Check sheet for the drawn part. Datum: minimum x, y, z corner. Units: mm. A direction names the side the tool comes from. Give positions to 0.01 mm unless a question says otherwise; leave off trailing zeros. Order: outer loops, then holes, each group sorted by start corner. A loop starts at its lowest first (then second) coordinate and runs counter-clockwise, first axis right, second up. Notation, with made-up numbers: M 61.5,-39.75 L 101.5,-39.75 A26 ccw 101.5,-25.75 Z; hole C -34,-39 d6. An arc over 180 degrees is marked long. Answer in a Markdown table with one row per item. Add a question column.
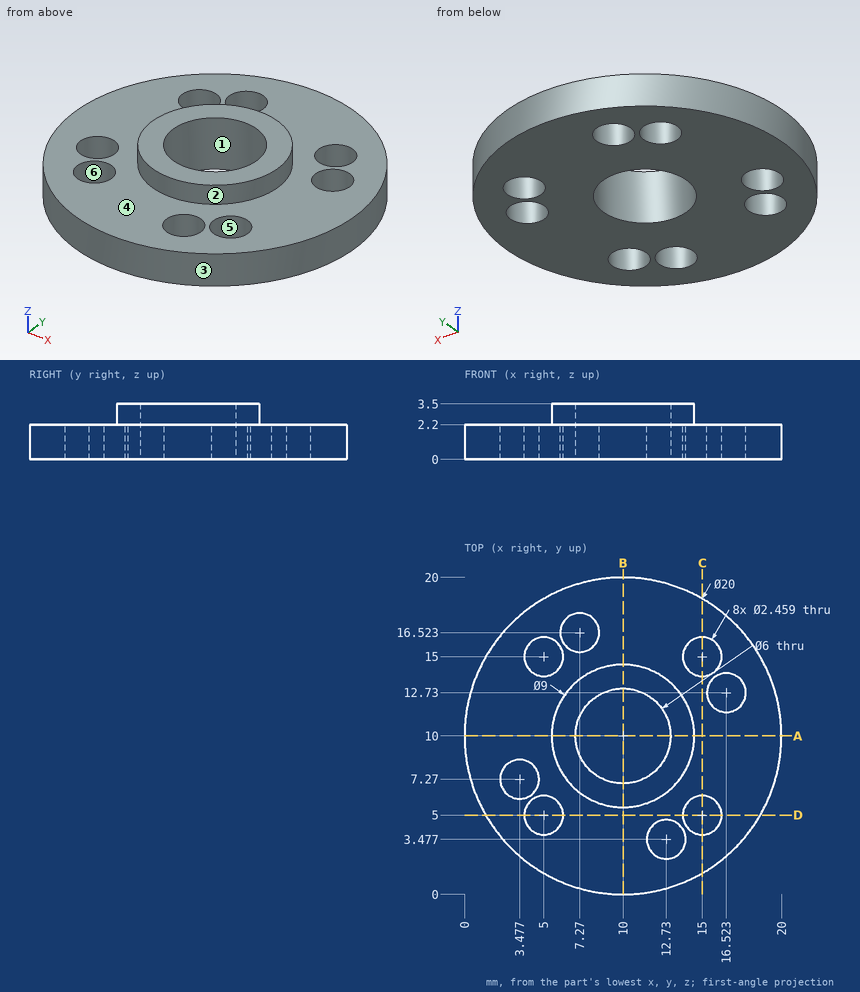
Q1. Go/stop test with flat-tipped pins: pin 1 (1.5 mm diameter, centred on x = 18, z = 1, fed in from +Y); pin 2 (1 mm diameter, centred on x = 12.5, z = 2, fed in from -Y); pin 3 (1.5 mm diameter, centred on x = 2, y = 15.5, fed in from -Z); pin 4 (12 mm diameter, centred on x = 18, y = 17, fed in from +Z). Record where each tip stops, or that it passes through.
Q2. Cross-section at C-C (x = 15). Record the boundary of the cut face in (y, z), and give its area (3 significant figures).
Q3. Draft check along X on the marked faces 3, 4, 5 and 6. Enter one of: pulls with the +X half, pulls with the -X half, needs draft (parallel to the pull), parting line crosses it, or undercut.
Q4. Tool access check on the marked faces 1 and 2. Record the directions out of +Z, -Z, +X, -X, +Y, -Y that give a thin tool (end or side, any length) a straight path to the whole face; none if there is none.
Q5. Thickness scan on probe 1 along X at (y, z) = (14.5, 2); probe 2 along Y at (x, z) = (10, 1.95); probe 3 along X at (y, z) = (7.75, 0.6) (1 decimal). Record the ranges inside material, lowest first.
Q6. Cross-section at A-A (y = 10). Record the boundary of the cut face in (x, z).
Values follow:
| question | item | result |
|---|---|---|
| 1 | pin 1 | y = 16.89 |
| 1 | pin 2 | y = 0.2 |
| 1 | pin 3 | z = 0 |
| 1 | pin 4 | z = 2.2 |
| 2 | outline | M 1.34,0 L 3.77,0 L 3.77,2.2 L 1.34,2.2 Z; M 6.23,0 L 13.77,0 L 13.77,2.2 L 6.23,2.2 Z; M 16.23,0 L 18.66,0 L 18.66,2.2 L 16.23,2.2 Z |
| 2 | area | 27.3 mm² |
| 3 | face 3 | parting line crosses it |
| 3 | face 4 | needs draft |
| 3 | face 5 | undercut |
| 3 | face 6 | undercut |
| 4 | face 1 | +Z, -Z |
| 4 | face 2 | +Z |
| 5 | probe 1 | 1.07 to 3.88, 6.12 to 13.88, 16.12 to 18.93 |
| 5 | probe 2 | 0 to 7, 13 to 20 |
| 5 | probe 3 | 0.3 to 2.3, 4.6 to 8, 12 to 19.7 |
| 6 | outline | M 0,0 L 7,0 L 7,3.5 L 5.5,3.5 L 5.5,2.2 L 0,2.2 Z; M 13,0 L 20,0 L 20,2.2 L 14.5,2.2 L 14.5,3.5 L 13,3.5 Z |
